Verification items for this drawing (mm, ordinates from the low corner). Give positions to 0.01 mm unless a question says otherwise; leave off trailing zeros. Order: outer loops, then holes, each group sorted by start corner. A loop starts at its lowest first (then second) coordinate and runs counter-clockwise, first axis right, second up. Notation, with made-up numbers: (-13, 40.25) -> (15, 40.25) arc R22 cw to (15, 57.25) -> close; hole circle Ø1 at (68.5, 5.25). An arc over 180 degrees is marked (long way). One line per question, with ' | ' between items.
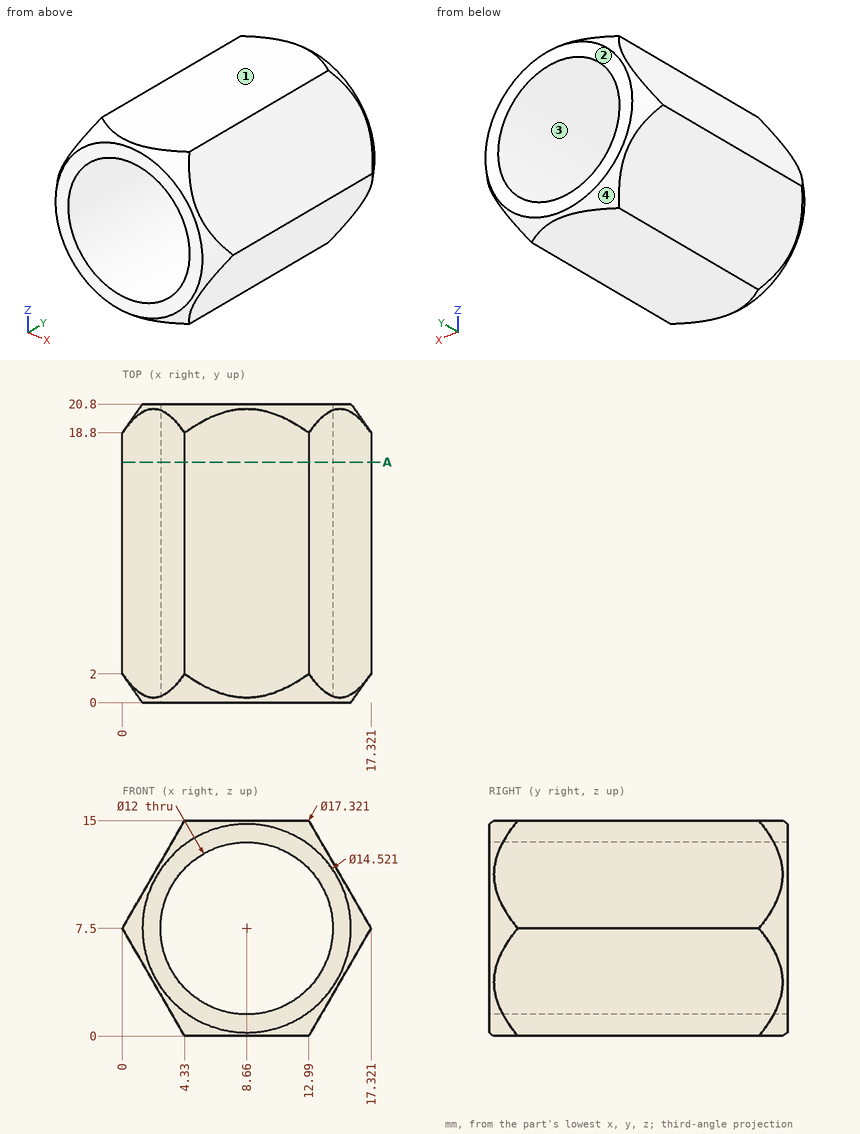
Q1. Mould release check, pull along Z, two halves, no side actions. Record for the marked faces 1, 2, 3 and 4: pulls with the +Z half, pulls with the -Z half, needs draft (parallel to the pull), parting line crosses it, or undercut.
Result sheet:
face 1: pulls with the +Z half | face 2: needs draft | face 3: undercut | face 4: parting line crosses it
Q2. Section check A-A (y = 16.75). Enter the section's corners in (x, z).
Result sheet:
outline: (0, 7.5) -> (4.33, 0) -> (12.99, 0) -> (17.32, 7.5) -> (12.99, 15) -> (4.33, 15) -> close; hole circle Ø12 at (8.66, 7.5)
Q3. Thickness scan on line 1 (Z direction, x = 11.75, y = 14.5) (1 decimal); line 2 (Z direction, x = 5.75, y = 10) (1 decimal); line 3 (X direction, y = 12.75, z = 3.25) (1 decimal). Record the ranges inside material, lowest first.
Result sheet:
line 1: z = 0 to 2.4, 12.6 to 15 | line 2: z = 0 to 2.3, 12.7 to 15 | line 3: x = 2.5 to 4.4, 12.9 to 14.9
Q4. Depth check by flat-ended pin: pin 1 Ø3 at (x, z) = (3, 12.5) entering from -Y; pin 2 Ø1.5 at (x, y) = (3.5, 3) entering from -Z. Enter the tip coordinate at first touch or a pass-through.
Result sheet:
pin 1: stops at y = 0 | pin 2: stops at z = 0.14
